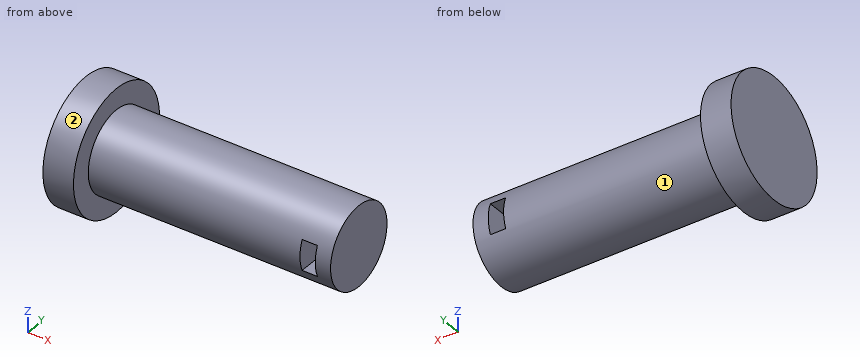
from build123d import *

# Parameters (mm, degrees)
SKETCH1_R               = 26.25
BOSS_EXTRUDE1_DEPTH     = 158.5
SKETCH2_R               = 40
BOSS_EXTRUDE2_DEPTH     = 20
CUT_EXTRUDE1_DEPTH      = 169.29215668
CUT_EXTRUDE1_DEPTH_BACK = 169.29215668
SKETCH3_W               = 10
SKETCH3_H               = 20


with BuildPart() as part:
    # Sketch1 → Boss-Extrude1 (new body)
    with BuildSketch(Plane(origin=(0, 0, 0), x_dir=(0, 0, -1), z_dir=(1, 0, 0))):
        Circle(SKETCH1_R)
    extrude(amount=BOSS_EXTRUDE1_DEPTH)

    # Sketch2 → Boss-Extrude2 (add)
    with BuildSketch(Plane.ZY):
        Circle(SKETCH2_R)
    extrude(amount=BOSS_EXTRUDE2_DEPTH)

    # Sketch3 → Cut-Extrude1 (cut, two sides: drawn at the far end of the back side and taken through both)
    with BuildSketch(Plane(origin=(0, 0, 0), x_dir=(1, 0, 0), z_dir=(0, 1, 0)).offset(-CUT_EXTRUDE1_DEPTH_BACK)):
        with Locations((143.5, 0)):
            Rectangle(SKETCH3_W, SKETCH3_H)
    extrude(amount=CUT_EXTRUDE1_DEPTH + CUT_EXTRUDE1_DEPTH_BACK, mode=Mode.SUBTRACT)


solid = part.part
Geometry: final body of the model. Coordinates: model frame, mm. Face numbers are marked on the shaded views. A direction names the side the tool comes from. Give positions to 0.01 mm unless a question says otherwise; leave off trailing zeros. Loops run counter-clockwise (first coordinate to the right, second up) from the corner with the lowest first, then second, coordinate; pieces in that order, holes last. Notation, with made-up numbers: (-10, 77) - (2, 77) arc R20 cw to (2, 108) - close; hole circle Ø1 at (-8.75, -21.75). An arc over 180 degrees is marked (long way). One line per question, with ' | ' between items. Start each with the question number.
(1) Contact query for flat-ended pins moving along their axis: pin 1 (6 mm diameter, centred on y = -26, z = 21, fed in from +X); pin 2 (10 mm diameter, centred on x = 2.5, z = 10, fed in from +Y); pin 3 (1 mm diameter, centred on x = 88, z = -7.5, fed in from -Y). Output: stop coordinate, or through.
(2) Section query D-D on z = -19.5. Return loops of the section in (x, y), then the cut area to 3 significant figures.
(3) Reachability of the marked faces 1 and 2 from +Z, -Z, +X, -X, +Y, -Y: full face, straight path, thin tool, end or side. Return the list, or none.
(4) Section query C-C on x = 142. Return loops of the section in (y, z), then the cut area to 3 significant figures.
(5) Section query B-B on y = 0. Return loops of the section in (x, z).
(6) Ray query, line 1 (X direction, y = -6, z = -3); line 2 (Z direction, x = 143.5, y = -23); line 3 (X direction, y = 25.5, z = 17). Return the intervals inside material, ascending. Write a range as from..to.
(7) Section query A-A on z = 0. Return loops of the section in (x, y).
The answers:
1) pin 1: x = 0 | pin 2: y = 39.6 | pin 3: y = -25.3
2) outline: (-20, -34.92) - (0, -34.92) - (0, -17.57) - (158.5, -17.57) - (158.5, 17.57) - (0, 17.57) - (0, 34.92) - (-20, 34.92) - close | area: 6,970 mm2
3) face 1: +X | face 2: +X, -X
4) outline: (-24.27, -10) arc R26.25 ccw to (24.27, -10) - close; (-24.27, 10) - (24.27, 10) arc R26.25 ccw to start | area: 1,140 mm2
5) outline: (-20, -40) - (0, -40) - (0, -26.25) - (158.5, -26.25) - (158.5, 26.25) - (0, 26.25) - (0, 40) - (-20, 40) - close; hole (138.5, -10) - (148.5, -10) - (148.5, 10) - (138.5, 10) - close
6) line 1: -20..138.5, 148.5..158.5 | line 2: -12.65..-10, 10..12.65 | line 3: -20..0
7) outline: (-20, -40) - (0, -40) - (0, -26.25) - (138.5, -26.25) - (138.5, 26.25) - (0, 26.25) - (0, 40) - (-20, 40) - close; (148.5, -26.25) - (158.5, -26.25) - (158.5, 26.25) - (148.5, 26.25) - close
